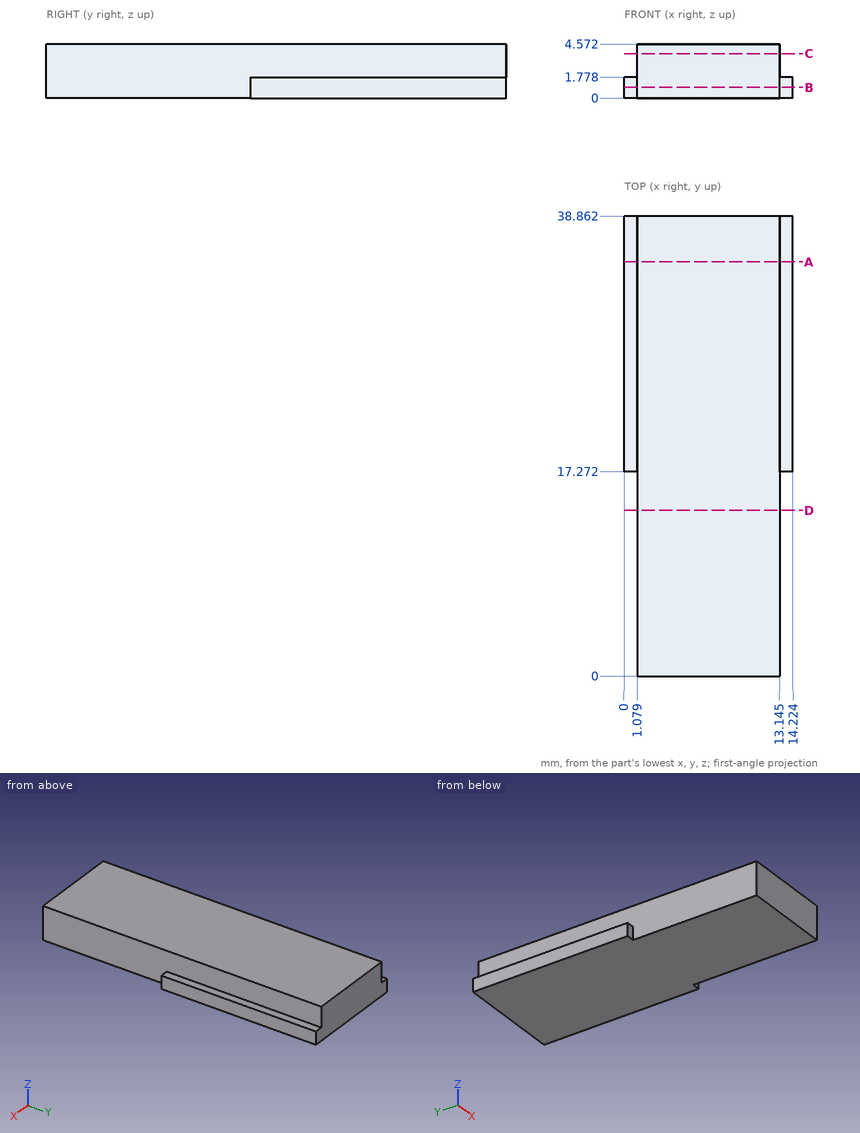
Here's the drawing with two shaded views (mm, measured from the low corner). I have some questions. Give positions to 0.01 mm unless a question says otherwise; leave off trailing zeros. Order: outer loops, then holes, each group sorted by start corner. A loop starts at its lowest first (then second) coordinate and runs counter-clockwise, first axis right, second up. Notation, with made-up numbers: (86.25, 73.25) - (98.25, 73.25) arc R6 cw to (98.25, 82.25) - close; hole circle Ø8 at (24, 29.25). An arc over 180 degrees is marked (long way). Use a Markdown table: item, result. Add a question column.
Q1. Please list where this line runs through material, in increasing order: line 1 along X through (y, z) = (9.5, 0.4) (1 decimal).
Q2. If we section it at A-A on y = 35: Write out the boundary of the cut face in (x, z) (1 decimal).
Q3. If we section it at B-B on z = 0.9: Write out the boundary of the cut face in (x, y) (1 decimal).
Q4. If we section it at D-D on y = 14: Write out the boundary of the cut face in (x, z) (1 decimal).
Q5. If we section it at C-C on z = 3.75: Write out the boundary of the cut face in (x, y) (1 decimal).
Q6. I'm going to push flat-ended pins straight in: pin 1 (0.5 mm diameter, centred on x = 0.5, z = 1, fed in from -Y); pin 2 (2 mm diameter, centred on x = 3.5, y = 11, fed in from -Z). Where does each tip first touch, or does it pass through?
Answers follow:
| question | item | result |
|---|---|---|
| 1 | line 1 | x = 1.1 to 13.1 |
| 2 | outline | (0, 0) - (14.2, 0) - (14.2, 1.8) - (13.1, 1.8) - (13.1, 4.6) - (1.1, 4.6) - (1.1, 1.8) - (0, 1.8) - close |
| 3 | outline | (0, 17.3) - (1.1, 17.3) - (1.1, 0) - (13.1, 0) - (13.1, 17.3) - (14.2, 17.3) - (14.2, 38.9) - (0, 38.9) - close |
| 4 | outline | (1.1, 0) - (13.1, 0) - (13.1, 4.6) - (1.1, 4.6) - close |
| 5 | outline | (1.1, 0) - (13.1, 0) - (13.1, 38.9) - (1.1, 38.9) - close |
| 6 | pin 1 | stops at y = 17.27 |
| 6 | pin 2 | stops at z = 0 |
